Autodesk Inventor part; units mm, degrees
ref_plane "YZ Plane" through (0, 0, 0) normal (1, 0, 0) x (0, 1, 0)
ref_plane "XZ Plane" through (0, 0, 0) normal (0, 1, 0) x (-1, 0, 0)
ref_plane "XY Plane" through (0, 0, 0) normal (0, 0, 1) x (1, 0, 0)
sketch "Sketch1" plane through (0, 0, 0) normal (0, 0, 1) x (1, 0, 0)
  line L0 (13.75, -9.25) -> (-13.75, -9.25)
  line L1 (-13.75, -9.25) -> (-13.75, 9.25)
  line L2 (-13.75, 9.25) -> (13.75, 9.25)
  line L3 (13.75, 9.25) -> (13.75, -9.25)
  line L4 (13.75, -9.25) -> (-13.75, 9.25) construction
  line L5 (-13.75, -9.25) -> (13.75, 9.25) construction
  line L6 (-16, 0) -> (16, 0) construction
  circle A0 centre (-16, 0) radius 4
  circle A1 centre (16, 0) radius 4
  line L7 (30, -1) -> (-30, -1)
  line L8 (-30, -1) -> (-30, 1)
  line L9 (-30, 1) -> (30, 1)
  line L10 (30, 1) -> (30, -1)
  line L11 (30, -1) -> (-30, 1) construction
  line L12 (-30, -1) -> (30, 1) construction
  line L13 (30, -6.5) -> (-30, -6.5)
  line L14 (-30, -6.5) -> (-30, 6.5)
  line L15 (-30, 6.5) -> (30, 6.5)
  line L16 (30, 6.5) -> (30, -6.5)
  line L17 (30, -6.5) -> (-30, 6.5) construction
  line L18 (-30, -6.5) -> (30, 6.5) construction
  line L19 (10, -5.5) -> (-10, -5.5) construction
  line L20 (-10, -5.5) -> (-10, 5.5) construction
  line L21 (-10, 5.5) -> (10, 5.5) construction
  line L22 (10, 5.5) -> (10, -5.5) construction
  line L23 (10, -5.5) -> (-10, 5.5) construction
  line L24 (-10, -5.5) -> (10, 5.5) construction
  circle A2 centre (-10, 5.5) radius 3
  circle A3 centre (10, 5.5) radius 3
  circle A4 centre (10, -5.5) radius 3
  circle A5 centre (-10, -5.5) radius 3
  line L25 (7, -9.25) -> (-7, -9.25)
  line L26 (-7, -9.25) -> (-7, 9.25)
  line L27 (-7, 9.25) -> (7, 9.25)
  line L28 (7, 9.25) -> (7, -9.25)
  line L29 (7, -9.25) -> (-7, 9.25) construction
  line L30 (-7, -9.25) -> (7, 9.25) construction
  line L31 (13, -9.25) -> (-13, -9.25)
  line L32 (-13, -9.25) -> (-13, 9.25)
  line L33 (-13, 9.25) -> (13, 9.25)
  line L34 (13, 9.25) -> (13, -9.25)
  line L35 (13, -9.25) -> (-13, 9.25) construction
  line L36 (-13, -9.25) -> (13, 9.25) construction
  point P0 (0, 0)
  point P1 (-19.873, -1)
  point P2 (-13.75, -6.5)
  point P3 (13.75, -6.5)
  point P4 (19.873, -1)
  point P5 (19.873, 1)
  point P6 (13.75, 6.5)
  point P7 (-13.75, 6.5)
  point P8 (-19.873, 1)
  point P9 (-13, -6.5)
  point P10 (-13, -5.5)
  point P11 (-7, -5.5)
  point P12 (7, -5.5)
  point P13 (13, -5.5)
  point P14 (13, -6.5)
  point P15 (13, 6.5)
  point P16 (13, 5.5)
  point P17 (7, 5.5)
  point P18 (-7, 5.5)
  point P19 (-13, 5.5)
  point P20 (-13, 6.5)
  dimension "d0" = 27.5
  dimension "d1" = 18.5
  dimension "d2" = 8
  dimension "d3" = 8
  dimension "d4" = 32
  dimension "d5" = 60
  dimension "d6" = 2
  dimension "d7" = 13
  dimension "d35" = 20
  dimension "d36" = 11
  dimension "d37" = 6
extrude "Extrusion1" add sketch "Sketch1" along normal blind 1.5875 contours L13 L34 A1 L3 | L3 A1 L7 L16 L13 | L0 L26 L13 L28 | A1 L34 L7 L3 | L3 L7 A1 | L13 L26 L7 L28 | A4 L28 L7 A1 L34 | L7 L34 L9 L3 | L3 L9 A1 L7 | A1 L7 L34 | A1 L9 L10 L7 | L9 L34 A1 L3 | L3 A1 L9 | L7 A1 L9 L34 | L7 L28 L9 A1 | L9 A1 L3 L15 L16 | L13 L1 A0 L32 | A5 L32 A0 L7 L26 | L7 L26 L9 L28 | A1 L34 L15 L3 | L9 A1 L34 | L9 L28 A3 L34 A1 | L13 L14 L7 A0 L1 | L7 A0 L9 L26 | L9 L26 L15 L28 | A0 L7 L1 | L1 L7 L32 A0 | L32 L7 A0 | L7 L32 L9 A0 | L9 A0 L32 A2 L26 | L7 A0 L9 L1 | L1 L9 L32 L7 | L7 L8 L9 A0 | L9 L32 A0 | L15 L26 L2 L28 | L9 A0 L1 | L1 A0 L32 L9 | L9 L14 L15 L1 A0 | A0 L1 L15 L32
fillet "Fillet2" radius 2 4 edges at (-30, 6.5, 0.7937) (-30, -6.5, 0.7937) (30, 6.5, 0.7937) (30, -6.5, 0.7937)
fillet "Fillet5" radius 1 8 edges at (-7, 9.25, 0.7937) (-7, -9.25, 0.7937) (-13, 6.5, 0.7937) (-13, -6.5, 0.7937) (13, -6.5, 0.7937) (13, 6.5, 0.7937) (7, 9.25, 0.7937) (7, -9.25, 0.7937)
sketch "Sketch3" plane through (0, 0, 1.5875) normal (0, 0, 1) x (1, 0, 0)
  point P0 (0, 0)
hole "Hole2" at (0, 0, 1.5875) direction (0, 0, -1) diameter 2.459 end through all
properties part number "Printhead Belt Retainer Cap" material "Aluminum 6061"
Model file for the job. Use its own axes, mm. A direction names the side the tool comes from. Coordinates: 2 decimals unless noted, no trailing zeros. Write each loop counter-clockwise with the first axis right and the second up, starting at its lowest first coordinate (ties: lowest second). Pieces come first, ordered by that corner, then holes. Notation, with made-up numbers: (8.5, -33.75) - (50.5, -33.75) arc R23 ccw to (50.5, -0.75) - close; hole circle Ø9 at (75.25, -20.5). An arc over 180 degrees is marked (long way). Use a Markdown table: item, result. Add a question column.
Item 1: 3-axis set-ups, long thin cutter, end or side, ignore diameter. For faces 4 (the face through (21, -6.5, 1)), 5 (the face through (13.301, 6.215, 0.805)), 6 (the face through (0.748, 0.976, 0.783)), 7 (the face through (-21, 6.5, 1)), 8 (the face through (13.285, -6.199, 0.805)): which of +Z, -Z, +X, -X, +Y, -Y reach the whole face in a straight line?
Item 2: Band-saw the part on B-B, the plane x = 0. Write the cut outline in (y, z).
Item 3: Band-saw the part on A-A, the plane y = 0. Write the cut outline in (x, z).
Item 4: Drill centre lines: line 1 along Y through (x, z) = (0, 0.65); line 2 along X through (y, z) = (5, 0.45); line 3 along X through (y, z) = (0, 0.5). Where is each one in solid material? Low to high.
Item 5: Band-saw the part on D-D, the plane y = -7.25. Write the cut outline in (x, z).
Item 6: Two-plate mould, pull along X, no slides. Class faces 1 (the face through (-13.301, -6.215, 0.805)), 2 (the face through (0, 9.25, 1)), 3 (the face through (-29.4, 5.93, 0.8)): pulls with the +X half, pulls with the -X half, needs draft (parallel to the pull), parting line crosses it, or undercut.
Item 7: Drop flat-ended pins along their axis: pin 1 (0.5 mm diameter, centred on y = 7.5, z = 1, fed in from +X); pin 2 (0.8 mm diameter, centred on x = 21.5, z = 1, fed in from -Y); pin 3 (0.5 mm diameter, centred on y = 6.5, z = 0.5, fed in from -X). Give the stop position or say it passes through.
A:
| question | item | result |
|---|---|---|
| 1 | face 4 | +Z, -Z, +X, -Y |
| 1 | face 5 | +Z, -Z, +Y |
| 1 | face 6 | +Z, -Z |
| 1 | face 7 | +Z, -Z, -X, +Y |
| 1 | face 8 | +Z, -Z, -Y |
| 2 | outline | (-9.25, 0) - (-1.23, 0) - (-1.23, 1.59) - (-9.25, 1.59) - close; (1.23, 0) - (9.25, 0) - (9.25, 1.59) - (1.23, 1.59) - close |
| 3 | outline | (-30, 0) - (-1.23, 0) - (-1.23, 1.59) - (-30, 1.59) - close; (1.23, 0) - (30, 0) - (30, 1.59) - (1.23, 1.59) - close |
| 4 | line 1 | y = -9.25 to -1.23, 1.23 to 9.25 |
| 4 | line 2 | x = -29.94 to -12.96, -7.04 to 7.04, 12.96 to 29.94 |
| 4 | line 3 | x = -30 to -1.23, 1.23 to 30 |
| 5 | outline | (-7, 0) - (7, 0) - (7, 1.59) - (-7, 1.59) - close |
| 6 | face 1 | undercut |
| 6 | face 2 | needs draft |
| 6 | face 3 | pulls with the -X half |
| 7 | pin 1 | stops at x = 7 |
| 7 | pin 2 | stops at y = -6.5 |
| 7 | pin 3 | stops at x = -28.97 |
